CAD build for the part. Positions are in the model's coordinates, mm. Face numbers are marked on the shaded views. Give positions to 0.01 mm unless a question says otherwise; leave off trailing zeros. Write each loop counter-clockwise with the first axis right and the second up, starting at its lowest first coordinate (ties: lowest second). Pieces come first, ordered by that corner, then holes. Notation, with made-up numbers: (-13.75, 51) - (14.25, 51) arc R25 ccw to (14.25, 79) - close; hole circle Ø11 at (36.25, 69.5). An arc over 180 degrees is marked (long way). Put each result on its own line as item: value. Start each with the question number.
1. Cut at D-D on z = 30. List the corners of the cut face in (x, y), and give its area (3 significant figures).
2. Wall check: line 1 (Y direction, x = -62, z = 7); line 2 (Y direction, x = 57.15, z = 2.75) (3 decimals); line 3 (Z direction, x = -46.5, y = 15). Give the ranges that are in metal, low to high.
3. Drop flat-ended pins along their axis: pin 1 (8 mm diameter, centred on x = 55.5, y = 13.5, fed in from -Z); pin 2 (8 mm diameter, centred on x = -68, y = 29.5, fed in from +Z); pin 3 (3 mm diameter, centred on x = 67.5, y = 26, fed in from +Z); pin 4 (3 mm diameter, centred on x = 64.5, y = -28, fed in from +Z). Give the stop position or say it passes through.
4. Cut at A-A on x = 57.15. List the corners of the cut face in (y, z) (1 decimal), and give its area (3 significant figures).
5. Cut at C-C on x = 0. List the corners of the cut face in (y, z).
6. Cut at B-B on y = 0. List the corners of the cut face in (x, z), and give its area (3 significant figures).
7. Mould opens along Z. For the marked faces 1, 2, 3 and 4 say: +Z half, -Z half, draft (parallel to the pull), parting line (faces both ways), or undercut.
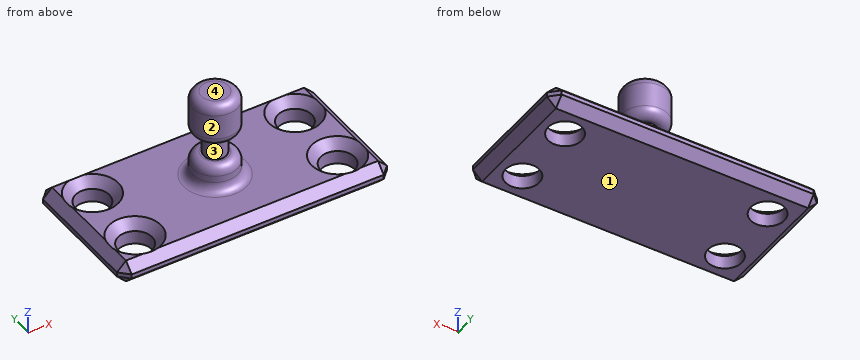
from build123d import *

# Parameters (mm, degrees)
F0_W         = 152.4
F0_H         = 76.2
F1_DEPTH     = 12.7
F2_R         = 9.525
F3_DEPTH     = 12.7
F4_W         = 12.7
F4_H         = 50.8
F6_W         = 7.62
F6_H         = 12.7
F8_R         = 5.08
F9_T1_DEPTH  = 6.4524666085
F9_T3_DEPTH  = 6.4524666085
F9_T5_DEPTH  = 6.4524666085
F9_T7_DEPTH  = 6.4524666085
F9_T9_DEPTH  = 6.4524666085
F9_T11_DEPTH = 6.4524666085
F9_T13_DEPTH = 6.4524666085
F9_T15_DEPTH = 6.4524666085
F9_T17_DEPTH = 102.3282991577
F9_T19_DEPTH = 178.5282991577
F9_T21_DEPTH = 38.8282991577


# Not quite as in the source:
# - a fillet or chamfer that OpenCascade refuses, or shapes differently, is made with other operations: its cross-section is extruded or revolved along the edge and cut away or added


with BuildPart() as f1:
    # F0 (on Top) → F1 (new body)
    with BuildSketch(Plane.XY):
        Rectangle(F0_W, F0_H)
    extrude(amount=F1_DEPTH)

    # F2 (on Top) → F3 (cut, symmetric)
    with BuildSketch(Plane.XY):
        with Locations((-57.15, 19.05)):
            Circle(F2_R)
        with Locations((57.15, 19.05)):
            Circle(F2_R)
        with Locations((57.15, -19.05)):
            Circle(F2_R)
        with Locations((-57.15, -19.05)):
            Circle(F2_R)
    extrude(amount=F3_DEPTH, both=True, mode=Mode.SUBTRACT)

    # F4 (on Front) → F5 (revolve)
    with BuildSketch(Plane.XZ):
        with Locations((6.35, 38.1)):
            Rectangle(F4_W, F4_H)
    revolve(axis=Axis((0, 0, 38.1), (0, 0, 1)))

    # F6 (on Front) → F7 (revolve, cut)
    with BuildSketch(Plane.XZ):
        with Locations((10.16, 32.980889082)):
            Rectangle(F6_W, F6_H)
    revolve(axis=Axis((0, 0, 12.7), (0, 0, 1)), mode=Mode.SUBTRACT)

    # F8
    f8_edges = [f1.edges().sort_by_distance(p)[0] for p in [
        (-12.7, 0, 12.7),
        (-12.7, 0, 63.5),
        (-12.7, 0, 26.630889),
        (-12.7, 0, 39.330889),
    ]]
    fillet(f8_edges, radius=F8_R)

    # F9: chamfer of 5.08 on 17 edges, made by hand

    # F9_s2 → F9_t1 (cut)
    with BuildSketch(Plane(origin=(38.9466666667, -38.9466666667, 38.9466666667), x_dir=(0.7071067812, 0.7071067812, 0), z_dir=(0.5773502692, -0.5773502692, 0.5773502692))):
        Polygon((26.9407683632, -32.1454703911), (30.5328708116, -38.3671743378), (23.3486659148, -38.3671743378), align=None)
    extrude(amount=F9_T1_DEPTH, mode=Mode.SUBTRACT)

    # F9_s4 → F9_t3 (cut)
    with BuildSketch(Plane(origin=(38.9466666667, 38.9466666667, 38.9466666667), x_dir=(-0.7071067812, 0.7071067812, 0), z_dir=(0.5773502692, 0.5773502692, 0.5773502692))):
        Polygon((-26.9407683632, -32.1454703911), (-30.5328708116, -38.3671743378), (-23.3486659148, -38.3671743378), align=None)
    extrude(amount=F9_T3_DEPTH, mode=Mode.SUBTRACT)

    # F9_s6 → F9_t5 (cut)
    with BuildSketch(Plane(origin=(-38.9466666667, -38.9466666667, 38.9466666667), x_dir=(0.7071067812, -0.7071067812, 0), z_dir=(-0.5773502692, -0.5773502692, 0.5773502692))):
        Polygon((-26.9407683632, -32.1454703911), (-23.3486659148, -38.3671743378), (-30.5328708116, -38.3671743378), align=None)
    extrude(amount=F9_T5_DEPTH, mode=Mode.SUBTRACT)

    # F9_s8 → F9_t7 (cut)
    with BuildSketch(Plane(origin=(-38.9466666667, 38.9466666667, 38.9466666667), x_dir=(-0.7071067812, -0.7071067812, 0), z_dir=(-0.5773502692, 0.5773502692, 0.5773502692))):
        Polygon((26.9407683632, -32.1454703911), (23.3486659148, -38.3671743378), (30.5328708116, -38.3671743378), align=None)
    extrude(amount=F9_T7_DEPTH, mode=Mode.SUBTRACT)

    # F9_s10 → F9_t9 (cut)
    with BuildSketch(Plane(origin=(-34.7133333333, -34.7133333333, -34.7133333333), x_dir=(0.7071067812, -0.7071067812, 0), z_dir=(-0.5773502692, -0.5773502692, -0.5773502692))):
        Polygon((-26.9407683632, 42.5149769689), (-23.3486659148, 48.7366809156), (-30.5328708116, 48.7366809156), align=None)
    extrude(amount=F9_T9_DEPTH, mode=Mode.SUBTRACT)

    # F9_s12 → F9_t11 (cut)
    with BuildSketch(Plane(origin=(34.7133333333, -34.7133333333, -34.7133333333), x_dir=(0.7071067812, 0.7071067812, 0), z_dir=(0.5773502692, -0.5773502692, -0.5773502692))):
        Polygon((26.9407683632, 42.5149769689), (30.5328708116, 48.7366809156), (23.3486659148, 48.7366809156), align=None)
    extrude(amount=F9_T11_DEPTH, mode=Mode.SUBTRACT)

    # F9_s14 → F9_t13 (cut)
    with BuildSketch(Plane(origin=(34.7133333333, 34.7133333333, -34.7133333333), x_dir=(-0.7071067812, 0.7071067812, 0), z_dir=(0.5773502692, 0.5773502692, -0.5773502692))):
        Polygon((-30.5328708116, 48.7366809156), (-26.9407683632, 42.5149769689), (-23.3486659148, 48.7366809156), align=None)
    extrude(amount=F9_T13_DEPTH, mode=Mode.SUBTRACT)

    # F9_s16 → F9_t15 (cut)
    with BuildSketch(Plane(origin=(-34.7133333333, 34.7133333333, -34.7133333333), x_dir=(-0.7071067812, -0.7071067812, 0), z_dir=(-0.5773502692, 0.5773502692, -0.5773502692))):
        Polygon((26.9407683632, 42.5149769689), (23.3486659148, 48.7366809156), (30.5328708116, 48.7366809156), align=None)
    extrude(amount=F9_T15_DEPTH, mode=Mode.SUBTRACT)

    # F9_s18 → F9_t17 (cut)
    with BuildSketch(Plane.XZ.offset(-51.1641495789)):
        Polygon((71.12, 12.7), (76.2, 7.62), (76.2, 12.7), align=None)
        Polygon((-71.12, 12.7), (-76.2, 7.62), (-76.2, 12.7), align=None)
        Polygon((-76.2, 5.08), (-71.12, 0), (-76.2, 0), align=None)
        Polygon((76.2, 5.08), (71.12, 0), (76.2, 0), align=None)
    extrude(amount=F9_T17_DEPTH, mode=Mode.SUBTRACT)

    # F9_s20 → F9_t19 (cut)
    with BuildSketch(Plane.YZ.offset(-89.2641495789)):
        Polygon((-33.02, 12.7), (-38.1, 7.62), (-38.1, 12.7), align=None)
        Polygon((33.02, 12.7), (38.1, 7.62), (38.1, 12.7), align=None)
        Polygon((-38.1, 5.08), (-33.02, 0), (-38.1, 0), align=None)
        Polygon((38.1, 5.08), (33.02, 0), (38.1, 0), align=None)
    extrude(amount=F9_T19_DEPTH, mode=Mode.SUBTRACT)

    # F9_s22 → F9_t21 (cut)
    with BuildSketch(Plane.XY.offset(-13.0641495789)):
        Polygon((-71.12, 38.1), (-76.2, 33.02), (-76.2, 38.1), align=None)
        Polygon((-71.12, -38.1), (-76.2, -33.02), (-76.2, -38.1), align=None)
        Polygon((76.2, -33.02), (71.12, -38.1), (76.2, -38.1), align=None)
        Polygon((76.2, 33.02), (71.12, 38.1), (76.2, 38.1), align=None)
    extrude(amount=F9_T21_DEPTH, mode=Mode.SUBTRACT)

    # F9_s23 → F9_t24 (revolve, cut)
    with BuildSketch(Plane.XZ.offset(19.05)):
        Polygon((-42.545, 12.7), (-47.625, 7.62), (-47.625, 12.7), align=None)
    revolve(axis=Axis((-57.15, -19.05, 12.7), (0, 0, 1)), mode=Mode.SUBTRACT)

    # F9_s25 → F9_t26 (revolve, cut)
    with BuildSketch(Plane.XZ.offset(19.05)):
        Polygon((71.755, 12.7), (66.675, 7.62), (66.675, 12.7), align=None)
    revolve(axis=Axis((57.15, -19.05, 12.7), (0, 0, 1)), mode=Mode.SUBTRACT)

    # F9_s27 → F9_t28 (revolve, cut)
    with BuildSketch(Plane.XZ.offset(-19.05)):
        Polygon((-42.545, 12.7), (-47.625, 7.62), (-47.625, 12.7), align=None)
    revolve(axis=Axis((-57.15, 19.05, 12.7), (0, 0, 1)), mode=Mode.SUBTRACT)

    # F9_s29 → F9_t30 (revolve, cut)
    with BuildSketch(Plane.XZ.offset(-19.05)):
        Polygon((71.755, 12.7), (66.675, 7.62), (66.675, 12.7), align=None)
    revolve(axis=Axis((57.15, 19.05, 12.7), (0, 0, 1)), mode=Mode.SUBTRACT)


solid = f1.part
Report:
1. outline: circle Ø12.7 at (0, 0)
1. area: 127 mm²
2. line 1: y = -38.1 to -27.25, -10.85 to 10.85, 27.25 to 38.1
2. line 2: y = -35.77 to -28.575, -9.525 to 9.525, 28.575 to 35.77
2. line 3: z = 0 to 9.49
3. pin 1: stops at z = 0
3. pin 2: stops at z = 12.7
3. pin 3: stops at z = 12.06
3. pin 4: stops at z = 11.18
4. outline: (-38.1, 5.1) - (-33, 0) - (-28.6, 0) - (-28.6, 7.6) - (-33.3, 12.4) - (-38.1, 7.6) - close; (-9.5, 0) - (9.5, 0) - (9.5, 7.6) - (4.4, 12.7) - (-4.4, 12.7) - (-9.5, 7.6) - close; (28.6, 0) - (33, 0) - (38.1, 5.1) - (38.1, 7.6) - (33.3, 12.4) - (28.6, 7.6) - close
4. area: 381 mm²
5. outline: (-38.1, 5.08) - (-33.02, 0) - (33.02, 0) - (38.1, 5.08) - (38.1, 7.62) - (33.02, 12.7) - (17.78, 12.7) arc R5.08 cw to (12.7, 17.78) - (12.7, 21.55) arc R5.08 ccw to (7.62, 26.63) - (6.35, 26.63) - (6.35, 39.33) - (7.62, 39.33) arc R5.08 ccw to (12.7, 44.41) - (12.7, 58.42) arc R5.08 ccw to (7.62, 63.5) - (-7.62, 63.5) arc R5.08 ccw to (-12.7, 58.42) - (-12.7, 44.41) arc R5.08 ccw to (-7.62, 39.33) - (-6.35, 39.33) - (-6.35, 26.63) - (-7.62, 26.63) arc R5.08 ccw to (-12.7, 21.55) - (-12.7, 17.78) arc R5.08 cw to (-17.78, 12.7) - (-33.02, 12.7) - (-38.1, 7.62) - close
6. outline: (-76.2, 5.08) - (-71.12, 0) - (71.12, 0) - (76.2, 5.08) - (76.2, 7.62) - (71.12, 12.7) - (17.78, 12.7) arc R5.08 cw to (12.7, 17.78) - (12.7, 21.55) arc R5.08 ccw to (7.62, 26.63) - (6.35, 26.63) - (6.35, 39.33) - (7.62, 39.33) arc R5.08 ccw to (12.7, 44.41) - (12.7, 58.42) arc R5.08 ccw to (7.62, 63.5) - (-7.62, 63.5) arc R5.08 ccw to (-12.7, 58.42) - (-12.7, 44.41) arc R5.08 ccw to (-7.62, 39.33) - (-6.35, 39.33) - (-6.35, 26.63) - (-7.62, 26.63) arc R5.08 ccw to (-12.7, 21.55) - (-12.7, 17.78) arc R5.08 cw to (-17.78, 12.7) - (-71.12, 12.7) - (-76.2, 7.62) - close
6. area: 2,990 mm²
7. face 1: -Z half
7. face 2: draft
7. face 3: undercut
7. face 4: +Z half
